Model file for the job. Use its own axes, mm. Face numbers are marked on the shaded views. A direction names the side the tool comes from. Round coordinates to 2 decimals unless told otherwise and drop trailing zeros. Order: outer loops, then holes, each group sorted by start corner. A loop starts at its lowest first (then second) coordinate and runs counter-clockwise, first axis right, second up. Notation, with made-up numbers: (46.25, -16.75) -> (60.25, -16.75) arc R14 ccw to (60.25, -5.75) -> close; hole circle Ø8 at (57, -28.5). An arc over 180 degrees is marked (long way). Put each result on its own line as item: value. Start each with the question number.
Q1. Probe L1, parallel to X at y = 14, z = 43; L2, parallel to X at y = 21.5, z = -23; L3, parallel to Y at x = -12.5, z = -15. List the from-to ranges inside material, lowest first.
Q2. Cut at B-B, the plane x = 13.5. State how many separate pieces and enclosed holes the cut face has, and give its area (3 significant figures).
Q3. Pull direction Z, two halves, no side cores. Call the marked faces 1, 2 and 3: released by +Z, released by -Z, zero draft, split by the parting line, or undercut.
Q4. Flat gauge pins, fed straight in: P1, Ø3, axis at x = 5, z = 43.5, coming from the +Y side; P2, Ø5, axis at x = 4, y = 22, coming from the +Z side; P3, Ø10, axis at x = -10, y = 14, coming from the +Z side; P4, Ø2, axis at y = 0.5, z = -33, coming from the +X side. Where does each tip first touch, or does it go through?
Q5. 3-axis set-ups, long thin cutter, end or side, ignore diameter. For the marked faces 4, 5, 6 and 7: which of +Z, -Z, +X, -X, +Y, -Y reach the whole face in a straight line?
Q6. Cut at A-A, the plane z = 18.5. List the corners of the cut face in (x, y), and give its area (3 significant figures).
from build123d import *
from OCP.BRepFilletAPI import BRepFilletAPI_MakeChamfer

# Parameters (mm, degrees)
SKETCH_1_W               = 52.4
SKETCH_1_H               = 115
EXTRUDE_1_DEPTH          = 7.5
CUT_EXTRUDE_1_DEPTH      = 64.631281615
CUT_EXTRUDE_1_DEPTH_BACK = 64.631281615
SKETCH_2_W               = 50
SKETCH_2_H               = 5
SKETCH_3_W               = 52.4
SKETCH_3_H               = 25
EXTRUDE_2_DEPTH          = 5
SKETCH_4_W               = 5
SKETCH_4_H               = 25
EXTRUDE_3_DEPTH          = 40
EXTRUDE_4_DEPTH          = 20
FILLET_1_R               = 10
SKETCH_7_R               = 5
CUT_EXTRUDE_2_DEPTH      = 20
CHAMFER_1_SIZE           = 1.2
CHAMFER_1_SIZE2          = 0.692820323
CHAMFER_2_SIZE           = 1.2
CHAMFER_2_SIZE2          = 0.692820323
CHAMFER_3_SIZE           = 1.2
CHAMFER_3_SIZE2          = 0.692820323
CHAMFER_4_SIZE           = 1.2
CHAMFER_4_SIZE2          = 0.692820323


with BuildPart() as part:
    # 스케치1 → 보스-돌출1 (new, symmetric)
    with BuildSketch(Plane(origin=(0, 0, 0), x_dir=(1, 0, 0), z_dir=(0, 1, 0))):
        Rectangle(SKETCH_1_W, SKETCH_1_H)
    extrude(amount=EXTRUDE_1_DEPTH, both=True)

    # 스케치2 → 컷-돌출1 (cut, two sides: drawn at the far end of the back side and taken through both)
    with BuildSketch(Plane(origin=(0, 0, 0), x_dir=(0, 0, -1), z_dir=(1, 0, 0)).offset(-CUT_EXTRUDE_1_DEPTH_BACK)):
        with Locations((27.5, 0)):
            Rectangle(SKETCH_2_W, SKETCH_2_H)
        with Locations((-27.5, 0)):
            Rectangle(SKETCH_2_W, SKETCH_2_H)
    extrude(amount=CUT_EXTRUDE_1_DEPTH + CUT_EXTRUDE_1_DEPTH_BACK, mode=Mode.SUBTRACT)

    # 스케치3 → 보스-돌출2 (add)
    with BuildSketch(Plane(origin=(0, 0, -57.5), x_dir=(-1, 0, 0), z_dir=(0, 0, -1))):
        with Locations((0, 20)):
            Rectangle(SKETCH_3_W, SKETCH_3_H)
    extrude(amount=-EXTRUDE_2_DEPTH)

    # 스케치4 → 보스-돌출3 (add)
    with BuildSketch(Plane.XY.offset(-52.5)):
        with Locations((-23.7, 20)):
            Rectangle(SKETCH_4_W, SKETCH_4_H)
        with Locations((23.7, 20)):
            Rectangle(SKETCH_4_W, SKETCH_4_H)
    extrude(amount=EXTRUDE_3_DEPTH)

    # 스케치5 → 보스-돌출4 (add)
    with BuildSketch(Plane.XY.offset(57.5)):
        with BuildLine():
            Line((-10.246950766, 32.5), (-26.2, 32.5))
            Line((-26.2, 32.5), (-26.2, 7.5))
            Line((-26.2, 7.5), (26.2, 7.5))
            Line((26.2, 7.5), (26.2, 32.5))
            Line((26.2, 32.5), (10.246950766, 32.5))
            ThreePointArc((10.246950766, 32.5), (0, 17.5), (-10.246950766, 32.5))
        make_face()
    extrude(amount=-EXTRUDE_4_DEPTH)

    # 필렛1
    fillet_1_edges = [part.edges().sort_by_distance(p)[0] for p in [
        (-10.246950766, 32.5, 47.5),
        (10.246950766, 32.5, 47.5),
    ]]
    fillet(fillet_1_edges, radius=FILLET_1_R)

    # 스케치7 → 컷-돌출2 (cut)
    with BuildSketch(Plane.XY.offset(57.5)):
        with Locations((-13.5, 14.5)):
            Circle(SKETCH_7_R)
        with Locations((13.5, 14.5)):
            Circle(SKETCH_7_R)
    extrude(amount=-CUT_EXTRUDE_2_DEPTH, mode=Mode.SUBTRACT)

    # 모따기1: one chamfer whose edges measure the first distance from different faces: ONE call of the kernel's chamfer builder (chamfer() names one face for all edges)
    chamfer_1_edges_1 = [part.edges().sort_by_distance(p)[0] for p in [
        (-23.162305899, 32.5, 57.5),
        (-14.148468751, 30.517837257, 57.5),
        (14.148468751, 30.517837257, 57.5),
        (0, -7.5, 57.5),
        (23.162305899, 32.5, 57.5),
        (0, 17.5, 57.5),
    ]]
    chamfer_1_side_1 = [part.faces().sort_by_distance(p)[0] for p in [
        (0, 9.670777652, 57.5),
    ]]
    chamfer_1_edges_2 = [part.edges().sort_by_distance(p)[0] for p in [
        (0, 17.5, 37.5),
        (-23.162305899, 32.5, 37.5),
        (-14.148468751, 30.517837257, 37.5),
        (14.148468751, 30.517837257, 37.5),
        (23.162305899, 32.5, 37.5),
    ]]
    chamfer_1_side_2 = [part.faces().sort_by_distance(p)[0] for p in [
        (-23.162305899, 31.919417534, 37.5),
    ]]
    chamfer_1_edges_3 = [part.edges().sort_by_distance(p)[0] for p in [
        (26.2, 32.5, -35),
        (26.2, -7.5, 0),
        (26.2, 32.5, 47.5),
    ]]
    chamfer_1_side_3 = [part.faces().sort_by_distance(p)[0] for p in [
        (26.2, 12.5, 56.282420434),
    ]]
    chamfer_1_edges_4 = [part.edges().sort_by_distance(p)[0] for p in [
        (-26.2, 32.5, -35),
        (-26.2, -7.5, 0),
        (-26.2, 32.5, 47.5),
    ]]
    chamfer_1_side_4 = [part.faces().sort_by_distance(p)[0] for p in [
        (-26.2, -6.282420434, 0),
    ]]
    chamfer_1_edges_5 = [part.edges().sort_by_distance(p)[0] for p in [
        (0, 32.5, -57.5),
        (0, -7.5, -57.5),
    ]]
    chamfer_1_side_5 = [part.faces().sort_by_distance(p)[0] for p in [
        (0, 12.5, -57.5),
    ]]
    chamfer_1_edges_6 = [part.edges().sort_by_distance(p)[0] for p in [
        (0, 32.5, -52.5),
    ]]
    chamfer_1_side_6 = [part.faces().sort_by_distance(p)[0] for p in [
        (0, 20, -52.5),
    ]]
    chamfer_1_edges_7 = [part.edges().sort_by_distance(p)[0] for p in [
        (-21.2, 32.5, -32.5),
    ]]
    chamfer_1_side_7 = [part.faces().sort_by_distance(p)[0] for p in [
        (-21.2, 20, -32.5),
    ]]
    chamfer_1_edges_8 = [part.edges().sort_by_distance(p)[0] for p in [
        (-23.7, 32.5, -12.5),
    ]]
    chamfer_1_side_8 = [part.faces().sort_by_distance(p)[0] for p in [
        (-23.7, 20, -12.5),
    ]]
    chamfer_1_edges_9 = [part.edges().sort_by_distance(p)[0] for p in [
        (21.2, 32.5, -32.5),
    ]]
    chamfer_1_side_9 = [part.faces().sort_by_distance(p)[0] for p in [
        (21.2, 20, -32.5),
    ]]
    chamfer_1_edges_10 = [part.edges().sort_by_distance(p)[0] for p in [
        (23.7, 32.5, -12.5),
    ]]
    chamfer_1_side_10 = [part.faces().sort_by_distance(p)[0] for p in [
        (23.7, 20, -12.5),
    ]]
    chamfer_1 = BRepFilletAPI_MakeChamfer(part.part.solid().wrapped)
    for e in chamfer_1_edges_1:
        chamfer_1.Add(CHAMFER_1_SIZE, CHAMFER_1_SIZE2, e.wrapped, chamfer_1_side_1[0].wrapped)  # the first distance lies on this face
    for e in chamfer_1_edges_2:
        chamfer_1.Add(CHAMFER_1_SIZE, CHAMFER_1_SIZE2, e.wrapped, chamfer_1_side_2[0].wrapped)  # the first distance lies on this face
    for e in chamfer_1_edges_3:
        chamfer_1.Add(CHAMFER_1_SIZE, CHAMFER_1_SIZE2, e.wrapped, chamfer_1_side_3[0].wrapped)  # the first distance lies on this face
    for e in chamfer_1_edges_4:
        chamfer_1.Add(CHAMFER_1_SIZE, CHAMFER_1_SIZE2, e.wrapped, chamfer_1_side_4[0].wrapped)  # the first distance lies on this face
    for e in chamfer_1_edges_5:
        chamfer_1.Add(CHAMFER_1_SIZE, CHAMFER_1_SIZE2, e.wrapped, chamfer_1_side_5[0].wrapped)  # the first distance lies on this face
    for e in chamfer_1_edges_6:
        chamfer_1.Add(CHAMFER_1_SIZE, CHAMFER_1_SIZE2, e.wrapped, chamfer_1_side_6[0].wrapped)  # the first distance lies on this face
    for e in chamfer_1_edges_7:
        chamfer_1.Add(CHAMFER_1_SIZE, CHAMFER_1_SIZE2, e.wrapped, chamfer_1_side_7[0].wrapped)  # the first distance lies on this face
    for e in chamfer_1_edges_8:
        chamfer_1.Add(CHAMFER_1_SIZE, CHAMFER_1_SIZE2, e.wrapped, chamfer_1_side_8[0].wrapped)  # the first distance lies on this face
    for e in chamfer_1_edges_9:
        chamfer_1.Add(CHAMFER_1_SIZE, CHAMFER_1_SIZE2, e.wrapped, chamfer_1_side_9[0].wrapped)  # the first distance lies on this face
    for e in chamfer_1_edges_10:
        chamfer_1.Add(CHAMFER_1_SIZE, CHAMFER_1_SIZE2, e.wrapped, chamfer_1_side_10[0].wrapped)  # the first distance lies on this face
    add(Compound.cast(chamfer_1.Shape()), mode=Mode.REPLACE)

    # 모따기2: one chamfer whose edges measure the first distance from different faces: ONE call of the kernel's chamfer builder (chamfer() names one face for all edges)
    chamfer_2_edges_1 = [part.edges().sort_by_distance(p)[0] for p in [
        (-18.5, 14.5, 37.5),
    ]]
    chamfer_2_side_1 = [part.faces().sort_by_distance(p)[0] for p in [
        (-25.624482841, 19.4, 37.5),
    ]]
    chamfer_2_edges_2 = [part.edges().sort_by_distance(p)[0] for p in [
        (-18.5, 14.5, 57.5),
    ]]
    chamfer_2_side_2 = [part.faces().sort_by_distance(p)[0] for p in [
        (0, 9.52416619, 57.5),
    ]]
    chamfer_2_edges_3 = [part.edges().sort_by_distance(p)[0] for p in [
        (8.5, 14.5, 37.5),
        (8.5, 14.5, 57.5),
    ]]
    chamfer_2_side_3 = [part.faces().sort_by_distance(p)[0] for p in [
        (8.5, 14.5, 47.5),
    ]]
    chamfer_2 = BRepFilletAPI_MakeChamfer(part.part.solid().wrapped)
    for e in chamfer_2_edges_1:
        chamfer_2.Add(CHAMFER_2_SIZE, CHAMFER_2_SIZE2, e.wrapped, chamfer_2_side_1[0].wrapped)  # the first distance lies on this face
    for e in chamfer_2_edges_2:
        chamfer_2.Add(CHAMFER_2_SIZE, CHAMFER_2_SIZE2, e.wrapped, chamfer_2_side_2[0].wrapped)  # the first distance lies on this face
    for e in chamfer_2_edges_3:
        chamfer_2.Add(CHAMFER_2_SIZE, CHAMFER_2_SIZE2, e.wrapped, chamfer_2_side_3[0].wrapped)  # the first distance lies on this face
    add(Compound.cast(chamfer_2.Shape()), mode=Mode.REPLACE)

    # 모따기3: one chamfer whose edges measure the first distance from different faces: ONE call of the kernel's chamfer builder (chamfer() names one face for all edges)
    chamfer_3_edges_1 = [part.edges().sort_by_distance(p)[0] for p in [
        (-26.2, 7.5, 12.5),
    ]]
    chamfer_3_side_1 = [part.faces().sort_by_distance(p)[0] for p in [
        (-26.2, 12.5, 56.290092566),
    ]]
    chamfer_3_edges_2 = [part.edges().sort_by_distance(p)[0] for p in [
        (26.2, 7.5, 12.5),
    ]]
    chamfer_3_side_2 = [part.faces().sort_by_distance(p)[0] for p in [
        (26.2, 12.5, 56.290092566),
    ]]
    chamfer_3 = BRepFilletAPI_MakeChamfer(part.part.solid().wrapped)
    for e in chamfer_3_edges_1:
        chamfer_3.Add(CHAMFER_3_SIZE, CHAMFER_3_SIZE2, e.wrapped, chamfer_3_side_1[0].wrapped)  # the first distance lies on this face
    for e in chamfer_3_edges_2:
        chamfer_3.Add(CHAMFER_3_SIZE, CHAMFER_3_SIZE2, e.wrapped, chamfer_3_side_2[0].wrapped)  # the first distance lies on this face
    add(Compound.cast(chamfer_3.Shape()), mode=Mode.REPLACE)

    # 모따기4: one chamfer whose edges measure the first distance from different faces: ONE call of the kernel's chamfer builder (chamfer() names one face for all edges)
    chamfer_4_edges_1 = [part.edges().sort_by_distance(p)[0] for p in [
        (26.2, 18.8, 37.5),
        (26.2, 18.8, -12.5),
    ]]
    chamfer_4_side_1 = [part.faces().sort_by_distance(p)[0] for p in [
        (26.2, 18.8, 38.709907434),
    ]]
    chamfer_4_edges_2 = [part.edges().sort_by_distance(p)[0] for p in [
        (-26.2, 18.8, 37.5),
        (-26.2, 18.8, -12.5),
    ]]
    chamfer_4_side_2 = [part.faces().sort_by_distance(p)[0] for p in [
        (-26.2, 18.8, -13.709907434),
    ]]
    chamfer_4_edges_3 = [part.edges().sort_by_distance(p)[0] for p in [
        (21.2, 19.4, -12.5),
    ]]
    chamfer_4_side_3 = [part.faces().sort_by_distance(p)[0] for p in [
        (21.2, 19.4, -32.5),
    ]]
    chamfer_4_edges_4 = [part.edges().sort_by_distance(p)[0] for p in [
        (-21.2, 19.4, -12.5),
    ]]
    chamfer_4_side_4 = [part.faces().sort_by_distance(p)[0] for p in [
        (-21.2, 19.4, -32.5),
    ]]
    chamfer_4 = BRepFilletAPI_MakeChamfer(part.part.solid().wrapped)
    for e in chamfer_4_edges_1:
        chamfer_4.Add(CHAMFER_4_SIZE, CHAMFER_4_SIZE2, e.wrapped, chamfer_4_side_1[0].wrapped)  # the first distance lies on this face
    for e in chamfer_4_edges_2:
        chamfer_4.Add(CHAMFER_4_SIZE, CHAMFER_4_SIZE2, e.wrapped, chamfer_4_side_2[0].wrapped)  # the first distance lies on this face
    for e in chamfer_4_edges_3:
        chamfer_4.Add(CHAMFER_4_SIZE, CHAMFER_4_SIZE2, e.wrapped, chamfer_4_side_3[0].wrapped)  # the first distance lies on this face
    for e in chamfer_4_edges_4:
        chamfer_4.Add(CHAMFER_4_SIZE, CHAMFER_4_SIZE2, e.wrapped, chamfer_4_side_4[0].wrapped)  # the first distance lies on this face
    add(Compound.cast(chamfer_4.Shape()), mode=Mode.REPLACE)


solid = part.part
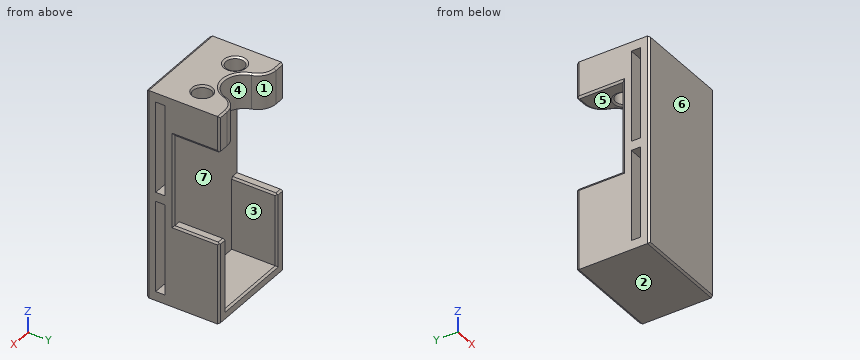
Ans:
1. L1: x = -26.2 to -18.47, -8.53 to 8.53, 18.47 to 26.2
1. L2: x = -26.2 to -21.2, 21.2 to 26.2
1. L3: y = -7.5 to -2.5, 2.5 to 7.5
2. separate pieces: 2
2. enclosed holes: 2
2. area: 1,600 mm^2
3. face 1: zero draft
3. face 2: released by -Z
3. face 3: undercut
4. P1: stops at y = 19.63
4. P2: stops at z = -52.5
4. P3: stops at z = 57.5
4. P4: passes through
5. face 4: +Z, +Y
5. face 5: +X, -X, +Y
5. face 6: +Z, -Z, +X, -X, -Y
5. face 7: +Y
6. outline: (-26.2, -6.3) -> (-25.51, -7.5) -> (25.51, -7.5) -> (26.2, -6.3) -> (26.2, -2.5) -> (-26.2, -2.5) -> close; (-26.2, 2.5) -> (26.2, 2.5) -> (26.2, 6.3) -> (25.51, 7.5) -> (-25.51, 7.5) -> (-26.2, 6.3) -> close
6. area: 522 mm^2
